Autodesk Inventor part; units mm, degrees
ref_plane "YZ Plane" through (0, 0, 0) normal (1, 0, 0) x (0, 1, 0)
ref_plane "XZ Plane" through (0, 0, 0) normal (0, 1, 0) x (-1, 0, 0)
ref_plane "XY Plane" through (0, 0, 0) normal (0, 0, 1) x (1, 0, 0)
sketch "Sketch1" plane through (0, 0, 0) normal (0, 0, 1) x (1, 0, 0)
  line L0 (-4.1, -22.5) -> (-4.1, -18)
  line L1 (-4.6, -18) -> (-6.8, -18)
  line L2 (-6.8, -18) -> (-6.8, -9.5)
  line L3 (-6.8, -9.5) -> (-4.5, -7.2)
  line L4 (-4.5, -7.2) -> (4.5, -7.2)
  line L5 (4.5, -7.2) -> (6.8, -9.5)
  line L6 (6.8, -9.5) -> (6.8, -18)
  line L7 (4.1, -18) -> (4.1, -22.5)
  line L8 (22.5, -4.1) -> (18, -4.1)
  line L9 (18, -4.6) -> (18, -6.8)
  line L10 (18, -6.8) -> (9.5, -6.8)
  line L11 (9.5, -6.8) -> (7.2, -4.5)
  line L12 (7.2, -4.5) -> (7.2, 4.5)
  line L13 (7.2, 4.5) -> (9.5, 6.8)
  line L14 (9.5, 6.8) -> (18, 6.8)
  line L15 (18, 4.1) -> (22.5, 4.1)
  line L16 (22.5, 22.5) -> (22.5, 4.4)
  line L17 (4.1, 22.5) -> (4.1, 18)
  line L18 (4.6, 18) -> (6.8, 18)
  line L19 (6.8, 18) -> (6.8, 9.5)
  line L20 (6.8, 9.5) -> (4.5, 7.2)
  line L21 (4.5, 7.2) -> (-4.5, 7.2)
  line L22 (-4.5, 7.2) -> (-6.8, 9.5)
  line L23 (-6.8, 9.5) -> (-6.8, 18)
  line L24 (-4.1, 18) -> (-4.1, 22.5)
  line L25 (-22.5, 22.5) -> (-4.4, 22.5)
  line L26 (-22.5, 4.1) -> (-18, 4.1)
  line L27 (-18, 6.8) -> (-9.5, 6.8)
  line L28 (-9.5, 6.8) -> (-7.2, 4.5)
  line L29 (-7.2, 4.5) -> (-7.2, -4.5)
  line L30 (-7.2, -4.5) -> (-9.5, -6.8)
  line L31 (-9.5, -6.8) -> (-18, -6.8)
  line L32 (-18, -6.8) -> (-18, -4.6)
  line L33 (-18, -4.1) -> (-22.5, -4.1)
  line L34 (-22.5, -22.5) -> (-22.5, -4.4)
  line L35 (-4.4, -22.5) -> (-22.5, -22.5)
  line L36 (-6.8, 18) -> (-4.1, 18)
  line L37 (4.1, 18) -> (4.6, 18)
  line L38 (-4.4, 22.5) -> (-3.1, 22.5)
  line L39 (3.1, 22.5) -> (22.5, 22.5)
  line L40 (18, 6.8) -> (18, 4.1)
  line L41 (18, -4.1) -> (18, -4.6)
  line L42 (22.5, 4.4) -> (22.5, 3.1)
  line L43 (22.5, -4.1) -> (22.5, -22.5)
  line L44 (6.8, -18) -> (4.1, -18)
  line L45 (-4.1, -18) -> (-4.6, -18)
  line L46 (22.5, -22.5) -> (4.1, -22.5)
  line L47 (-4.1, -22.5) -> (-4.4, -22.5)
  line L48 (-22.5, -4.4) -> (-22.5, -3.1)
  line L49 (-22.5, 3.1) -> (-22.5, 22.5)
  line L50 (-18, -4.6) -> (-18, -4.1)
  line L51 (-18, 4.1) -> (-18, 6.8)
  line L52 (-24.5, 24.5) -> (24.5, 24.5)
  line L53 (24.5, 24.5) -> (24.5, -24.5)
  line L54 (24.5, -24.5) -> (-24.5, -24.5)
  line L55 (-24.5, -24.5) -> (-24.5, 24.5)
  line L56 (-22.5, 3.1) -> (-17, 3.1)
  line L57 (-17, 5.8) -> (-9.5, 5.8)
  line L58 (-17, 3.1) -> (-17, 5.8)
  line L59 (-8.2, 4.5) -> (-8.2, 0)
  line L60 (-8.2, 4.5) -> (-9.5, 5.8)
  line L61 (-8.2, 4.5) -> (-5.6544, 4.5) construction
  line L62 (-24.5, 0) -> (0, 0)
  line L63 (-22.5, -3.1) -> (-17, -3.1)
  line L64 (-17, -3.1) -> (-17, -5.8)
  line L65 (-17, -5.8) -> (-9.5, -5.8)
  line L66 (-8.2, -4.5) -> (-8.2, 0)
  line L67 (-8.2, -4.5) -> (-9.5, -5.8)
  line L68 (-5.8, -17) -> (-5.8, -9.5)
  line L69 (-4.5, -8.2) -> (-5.8, -9.5)
  line L70 (-4.5, -8.2) -> (0, -8.2)
  line L71 (4.5, -8.2) -> (0, -8.2)
  line L72 (4.5, -8.2) -> (5.8, -9.5)
  line L73 (5.8, -17) -> (5.8, -9.5)
  line L74 (3.1, -17) -> (5.8, -17)
  line L75 (3.1, -22.5) -> (3.1, -17)
  line L76 (-3.1, -17) -> (-5.8, -17)
  line L77 (-3.1, -22.5) -> (-3.1, -17)
  line L78 (17, -5.8) -> (9.5, -5.8)
  line L79 (8.2, -4.5) -> (9.5, -5.8)
  line L80 (8.2, -4.5) -> (8.2, 0)
  line L81 (8.2, 4.5) -> (8.2, 0)
  line L82 (8.2, 4.5) -> (9.5, 5.8)
  line L83 (17, 5.8) -> (9.5, 5.8)
  line L84 (17, 3.1) -> (17, 5.8)
  line L85 (22.5, 3.1) -> (17, 3.1)
  line L86 (17, -3.1) -> (17, -5.8)
  line L87 (22.5, -3.1) -> (17, -3.1)
  line L88 (5.8, 17) -> (5.8, 9.5)
  line L89 (4.5, 8.2) -> (5.8, 9.5)
  line L90 (4.5, 8.2) -> (0, 8.2)
  line L91 (-4.5, 8.2) -> (0, 8.2)
  line L92 (-4.5, 8.2) -> (-5.8, 9.5)
  line L93 (-5.8, 17) -> (-5.8, 9.5)
  line L94 (-3.1, 17) -> (-5.8, 17)
  line L95 (-3.1, 22.5) -> (-3.1, 17)
  line L96 (3.1, 17) -> (5.8, 17)
  line L97 (3.1, 22.5) -> (3.1, 17)
  line L98 (22.5, -4.1) -> (22.5, -3.1)
  line L99 (4.1, -22.5) -> (3.1, -22.5)
  line L100 (-3.1, -22.5) -> (-4.1, -22.5)
  dimension "d7" = 45
  dimension "d8" = 49
  dimension "d9" = 49
  dimension "d11" = 24.5
  dimension "d12" = 24.5
  dimension "d13" = 1
  dimension "d14" = 1
  dimension "d15" = 1
  dimension "d16" = 135
  dimension "d17" = 4.5
  dimension "d20" = 360
extrude "Extrusion3" add sketch "Sketch1" along normal blind 20 contours L55 L52 L53 L54 | L0 L45 L1 L2 L3 L4 L5 L6 L44 L7 L99 L75 L74 L73 L72 L71 L70 L69 L68 L76 L77 L100 | L48 L63 L64 L65 L67 L66 L62 L29 L30 L31 L32 L50 L33 | L62 L59 L60 L57 L58 L56 L49 L26 L51 L27 L28 L29 | L8 L41 L9 L10 L11 L12 L13 L14 L40 L15 L42 L85 L84 L83 L82 L81 L80 L79 L78 L86 L87 L98 | L38 L95 L94 L93 L92 L91 L90 L89 L88 L96 L97 L39 L17 L37 L18 L19 L20 L21 L22 L23 L36 L24
sketch "Sketch3" plane through (0, 0, 0) normal (0, 0, -1) x (-1, 0, 0)
  line L0 (24.5, -24.5) -> (24.5, 24.5)
  line L1 (24.5, 24.5) -> (-24.5, 24.5)
  line L2 (-24.5, 24.5) -> (-24.5, -24.5)
  line L3 (-24.5, -24.5) -> (24.5, -24.5)
  line L4 (30, 30) -> (-90, 30)
  line L5 (-40, -30) -> (30, -30)
  line L6 (30, -30) -> (30, 30)
  line L7 (-90, -101.9604) -> (-40, -101.9604)
  line L8 (-40, -101.9604) -> (-40, -30)
  line L9 (-90, 30) -> (-90, -101.9604)
  point P0 (0, 0)
  dimension "d25" = 60
  dimension "d26" = 5.5
  dimension "d27" = 49
  dimension "d28" = 5.5
  dimension "d32" = 120
extrude "Extrusion4" add sketch "Sketch3" against normal blind 20
sketch "Sketch4" plane through (0, 0, 20) normal (0, 0, 1) x (1, 0, 0)
  circle A0 centre (65, -71.4443) radius 14.5
  line L0 (40, -101.9604) -> (90, -101.9604)
  line L1 (40, -30) -> (40, -101.9604)
  point P0 (0, 0)
  dimension "d33" = 29
  dimension "d34" = 50
  dimension "d35" = 25
extrude "Extrusion5" cut sketch "Sketch4" against normal up to next
sketch "Sketch5" plane through (40, -101.9604, 0) normal (0, -1, 0) x (1, 0, 0)
  line L0 (0, 20) -> (50, 20)
  line L1 (-70, 20) -> (0, 20)
  line L2 (-70, 0) -> (-70, 20)
  line L3 (0, 0) -> (-70, 0)
  line L4 (50, 0) -> (0, 0)
  line L5 (50, 0) -> (50, 20)
  circle A0 centre (34, 10) radius 4
  circle A1 centre (18, 10) radius 4
  line L6 (50, 0) -> (0, 0)
  line L7 (50, 0) -> (50, 20)
  line L8 (0, 20) -> (50, 20)
  line L9 (0, 0) -> (0, 20)
  point P0 (-40, 0)
  dimension "d38" = 8
  dimension "d39" = 8
  dimension "d40" = 16
  dimension "d41" = 20
  dimension "d42" = 10
  dimension "d43" = 10
  dimension "d44" = 32
extrude "Extrusion6" cut sketch "Sketch5" against normal blind 5 contours A0 | A1
equation "\"d9\" = d8"
equation "\"d11\" = 0.5 * d8"
equation "\"d12\" = d11"
equation "\"d26\" = d28"
equation "\"d28\" = -0.5 * d27 + 0.5 * d25"
equation "\"d35\" = 0.5 * d34"
equation "\"d39\" = d38"
equation "\"d42\" = 0.5 * d41"
equation "\"d43\" = d42"
equation "\"d44\" = d40 + 2 * d39"
properties part number "TrackPowerJoint" material "Aluminum-6061"
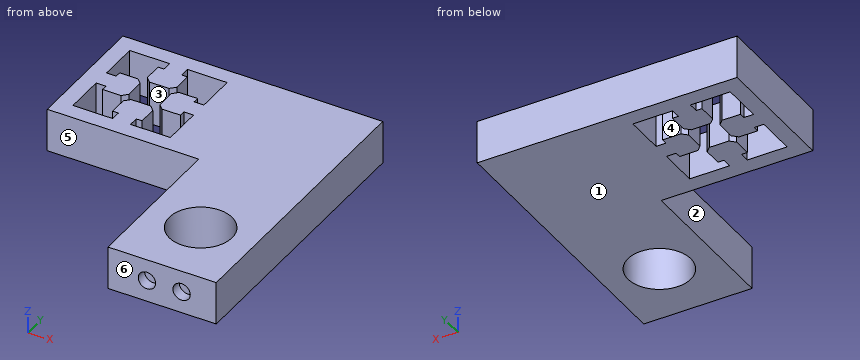
For this review, take the finished solid that the model builds, in its own axes (mm). Face numbers are marked on the shaded views. A direction names the side the tool comes from. Give positions to 0.01 mm unless a question says otherwise; leave off trailing zeros. Loops run counter-clockwise (first coordinate to the right, second up) from the corner with the lowest first, then second, coordinate; pieces in that order, holes last. Notation, with made-up numbers: M 58.25,72 L 66.25,72 A18 ccw 66.25,80 Z; hole C -32.75,-28.5 d3. An arc over 180 degrees is marked long. Put each result on its own line as item: value. Start each with the question number.
(1) Add section C-C, the plane y = -46. Write out the cut boundary in (x, z).
(2) Wall thickness on L1, parallel to Y at x = 15.5, z = 17.5; L2, parallel to X at y = -4.5, z = 19.25; L3, parallel to Z at x = 58, y = -98: over which ranges is each line inside the solid? List them lowest first.
(3) Add section A-A, the plane x = 65. Write out the cut boundary in (y, z).
(4) Add section B-B, the plane z = 12. Give the number of separate pieces and of enclosed holes in the cut face, then the cut area to 3 significant figures.
(5) Machinability: for the marked faces 4, 5 and 6, which of the approach directions +Z, -Z, +X, -X, +Y, -Y give a long, thin tool a straight path to every point of the face, cutting with its end or side? Answer none if there is none.
(6) The part is to be moulded in two halves that separate along X. For the marked faces 1, 2 and 3, say which applies: +X half, -X half, draft (parallel to the pull), parting line (faces both ways), or undercut.
(7) For pin 1 (4 mm diameter, centred on x = 64, y = 16.5, fed in from -Z); pin 2 (6 mm diameter, centred on y = -58.5, z = 7.5, fed in from -X); pin 3 (2 mm diameter, centred on x = 5.5, z = 5.5, fed in from -Y), all flat-tipped, find the tip position at first contact; note any pin that passes through.
Result:
1. outline: M 40,0 L 90,0 L 90,20 L 40,20 Z
2. L1: y = -30 to -22.5, -6.8 to 6.8, 22.5 to 30
2. L2: x = -30 to -22.5, -18 to -7.2, 7.2 to 18, 22.5 to 90
2. L3: z = 0 to 6, 14 to 20
3. outline: M -101.96,0 L -85.94,0 L -85.94,20 L -101.96,20 Z; M -56.94,0 L 30,0 L 30,20 L -56.94,20 Z
4. separate pieces: 1
4. enclosed holes: 2
4. area: 8,760 mm^2
5. face 4: +Z, -Z
5. face 5: +Z, -Z, -X, -Y
5. face 6: +Z, -Z, +X, -X, -Y
6. face 1: draft
6. face 2: -X half
6. face 3: undercut
7. pin 1: stops at z = 0
7. pin 2: stops at x = 40
7. pin 3: stops at y = -30
